```python
from build123d import *

# Parameters (mm, degrees)
SKETCH1_W           = 533.4
SKETCH1_H           = 508
SKETCH1_R           = 12.7
BOSS_EXTRUDE1_DEPTH = 152.4
BOSS_EXTRUDE2_DEPTH = 660.4
SKETCH4_OUTSIDE_W   = 729.384
SKETCH4_OUTSIDE_H   = 1034.184
CUT_EXTRUDE1_DEPTH  = 660.4
BOSS_EXTRUDE3_DEPTH = 50.8
SKETCH7_OUTSIDE_W   = 754.784
SKETCH7_OUTSIDE_H   = 1147.193
CUT_EXTRUDE2_DEPTH  = 254
CUT_EXTRUDE3_DEPTH  = 508


with BuildPart() as part:
    # Sketch1 → Boss-Extrude1 (new body)
    with BuildSketch(Plane(origin=(0, 0, 0), x_dir=(1, 0, 0), z_dir=(0, 1, 0))):
        Rectangle(SKETCH1_W, SKETCH1_H)
        with Locations(Location((-95.25, -130.175, 0), (0, 0, 90))):
            Circle(SKETCH1_R, mode=Mode.SUBTRACT)
        with Locations(Location((-95.25, 0, 0), (0, 0, 90))):
            Circle(SKETCH1_R, mode=Mode.SUBTRACT)
        with Locations(Location((-95.25, 130.175, 0), (0, 0, 90))):
            Circle(SKETCH1_R, mode=Mode.SUBTRACT)
        with Locations(Location((95.25, -130.175, 0), (0, 0, 90))):
            Circle(SKETCH1_R, mode=Mode.SUBTRACT)
        with Locations(Location((95.25, 0, 0), (0, 0, 90))):
            Circle(SKETCH1_R, mode=Mode.SUBTRACT)
        with Locations(Location((95.25, 130.175, 0), (0, 0, 90))):
            Circle(SKETCH1_R, mode=Mode.SUBTRACT)
    extrude(amount=BOSS_EXTRUDE1_DEPTH)

    # Sketch3 → Boss-Extrude2 (add)
    with BuildSketch(Plane(origin=(0, 152.4, 0), x_dir=(1, 0, 0), z_dir=(0, 1, 0))):
        Polygon((-266.7, 254), (-266.7, -254), (-165.1, -254), (165.1, -254), (266.7, -254), (266.7, 254), align=None)
    extrude(amount=BOSS_EXTRUDE2_DEPTH)

    # Sketch4 outside → Cut-Extrude1 (cut)
    with BuildSketch(Plane(origin=(266.7, 0, 0), x_dir=(0, 0, -1), z_dir=(1, 0, 0))):
        with Locations((0, 406.4)):
            Rectangle(SKETCH4_OUTSIDE_W, SKETCH4_OUTSIDE_H)
        with BuildLine():
            Line((254, 669.23901778), (254, 812.8))
            Line((254, 812.8), (228.6, 812.8))
            Line((228.6, 812.8), (31.606344145, 168.462784922))
            Line((31.606344145, 168.462784922), (-254, 168.462784922))
            ThreePointArc((-254, 168.462784922), (-243.936587472, 127.409322416), (-202.883124967, 117.345909888))
            Line((-202.883124967, 117.345909888), (-165.988990497, 0))
            Line((-165.988990497, 0), (165.353024922, 0))
            Line((165.353024922, 0), (228.6, 108.732858548))
            Line((228.6, 108.732858548), (254, 669.23901778))
        make_face(mode=Mode.SUBTRACT)
    extrude(amount=-CUT_EXTRUDE1_DEPTH, mode=Mode.SUBTRACT)

    # Sketch6 → Boss-Extrude3 (add)
    with BuildSketch(Plane.ZY.offset(266.7)):
        with BuildLine():
            Line((254, 168.462784922), (-31.606344145, 168.462784922))
            Line((-31.606344145, 168.462784922), (-93.174683572, 369.843749152))
            ThreePointArc((-93.174683572, 369.843749152), (37.15276036, 257.574854495), (204.490495991, 217.72978475))
            ThreePointArc((204.490495991, 217.72978475), (239.484222443, 203.385658011), (254, 168.462784922))
        make_face()
    boss_extrude3 = extrude(amount=-BOSS_EXTRUDE3_DEPTH)

    # Mirror1: Boss-Extrude3 across plane
    add(boss_extrude3.mirror(Plane.ZY))

    # Sketch7 outside → Cut-Extrude2 (cut)
    with BuildSketch(Plane(origin=(0, 5.563381647, 18.197001427), x_dir=(1, 0, 0), z_dir=(0, 0.29237170472274066, 0.9563047559630343))):
        with Locations((0, 388.6425)):
            Rectangle(SKETCH7_OUTSIDE_W, SKETCH7_OUTSIDE_H)
        with BuildLine():
            Line((-266.7, 380.92497735), (-209.55, 609.52497735))
            ThreePointArc((-209.55, 609.52497735), (-188.66895271, 653.395441882), (-152.4, 685.72497735))
            ThreePointArc((-152.4, 685.72497735), (-95.710918301, 736.501940936), (-63.5, 805.454161765))
            ThreePointArc((-63.5, 805.454161765), (-45.688148209, 833.291148022), (-14.465061194, 844.120677346))
            Line((-14.465061194, 844.120677346), (14.465061194, 844.120677346))
            ThreePointArc((14.465061194, 844.120677346), (45.688148209, 833.291148022), (63.5, 805.454161765))
            ThreePointArc((63.5, 805.454161765), (95.710918301, 736.501940936), (152.4, 685.72497735))
            ThreePointArc((152.4, 685.72497735), (188.66895271, 653.395441882), (209.55, 609.52497735))
            Line((209.55, 609.52497735), (266.7, 380.92497735))
            Line((266.7, 380.92497735), (266.7, -48.530484117))
            Line((266.7, -48.530484117), (-266.7, -48.530484117))
            Line((-266.7, -48.530484117), (-266.7, 380.92497735))
        make_face(mode=Mode.SUBTRACT)
    extrude(amount=-CUT_EXTRUDE2_DEPTH, mode=Mode.SUBTRACT)

    # Sketch10 → Cut-Extrude3 (cut)
    with BuildSketch(Plane.XY.offset(254)):
        with BuildLine():
            Line((-266.7, 168.462784922), (-387.417771375, 168.462784922))
            Line((-387.417771375, 168.462784922), (-387.417771375, 0))
            Line((-387.417771375, 0), (-155.638931275, 0))
            ThreePointArc((-155.638931275, 0), (-169.876966254, 49.659931769), (-208.265044728, 84.231392461))
            ThreePointArc((-208.265044728, 84.231392461), (-248.469302502, 118.725084742), (-266.7, 168.462784922))
        make_face()
        with BuildLine():
            Line((387.417771375, 0), (155.638931275, 0))
            ThreePointArc((155.638931275, 0), (169.876966254, 49.659931769), (208.265044728, 84.231392461))
            ThreePointArc((208.265044728, 84.231392461), (248.469302502, 118.725084742), (266.7, 168.462784922))
            Line((266.7, 168.462784922), (387.417771375, 168.462784922))
            Line((387.417771375, 168.462784922), (387.417771375, 0))
        make_face()
    extrude(amount=-CUT_EXTRUDE3_DEPTH, mode=Mode.SUBTRACT)


solid = part.part
```
Design review of the part built by this model. Coordinates are the model's own, in mm. A direction names the side the tool comes from. Give positions to 0.01 mm unless a question says otherwise; leave off trailing zeros. Order: outer loops, then holes, each group sorted by start corner. A loop starts at its lowest first (then second) coordinate and runs counter-clockwise, first axis right, second up. Notation, with made-up numbers: (10, 24.25) -> (24, 24.25) arc R21 cw to (24, 58.25) -> close; hole circle Ø8 at (-3, -1). An arc over 180 degrees is marked (long way). Write each question's results on one line, items separated by ' | '. Start each with the question number.
Q1. Add section C-C on z = 0. Give the boundary of the cut face in (x, y).
Q2. Wall thickness on L1, parallel to X at y = 48, z = 0; L2, parallel to Z at x = 95.25, y = 60.5 (3 decimals); L3, parallel to Z at x = -95.25, y = 50.5 (3 decimals): over which ranges is each line inside the solid? List them lowest first. Write a range as from..to.
Q3. Add section A-A on y = 49. Give the boundary of the cut face in (x, z) (3 decimals).
Q4. Add section D-D on y = 308. Give the boundary of the cut face in (x, z), and give its area (3 significant figures).
Q5. Mouldability with a two-part tool opening along Z and no side actions: class faces 1 (the flat face through (215.9, 225, 56)), 2 (the flat face through (-95, 152.4, -130)), 3 (the flat face through (-0.203, 808.972, -241.122)) as +Z half, -Z half, draft (parallel to the pull), parting line (faces both ways), or undercut.
Q6. Machinability: for faces 4 (the flat face through (95, 152.4, -130)), 5 (the cylindrical face through (-248.04, 118.11, 14.74)), which of the approach directions +Z, -Z, +X, -X, +Y, -Y give a long, thin tool a straight path to every point of the face, cutting with its end or side? Answer none if there is none.
Q7. Add section B-B on x = -95.25. Give the boundary of the cut face in (y, z) (3 decimals).
Q8. For pin 1 (6 mm diameter, centred on x = 177.5, y = 561, fed in from -Z); pin 2 (15 mm diameter, centred on x = -95.25, z = 130.175, fed in from -Y); pin 3 (15 mm diameter, centred on x = 95.25, z = 130.175, fed in from +Y), all flat-tipped, find the tip position at first contact; note any pin that passes through.
Found:
1) outline: (-266.7, 168.46) arc R104.93 ccw to (-208.27, 84.23) arc R93.72 cw to (-155.64, 0) -> (-107.95, 0) -> (-107.95, 152.4) -> (-82.55, 152.4) -> (-82.55, 0) -> (82.55, 0) -> (82.55, 152.4) -> (107.95, 152.4) -> (107.95, 0) -> (155.64, 0) arc R93.72 cw to (208.27, 84.23) arc R104.93 ccw to (266.7, 168.46) -> (266.7, 279.43) -> (215.9, 279.43) -> (215.9, 168.46) -> (-215.9, 168.46) -> (-215.9, 279.43) -> (-266.7, 279.43) -> close
2) L1: x = -168.86..-107.95, -82.55..82.55, 107.95..168.86 | L2: z = -200.544..-142.875, -117.475..-12.7, 12.7..117.475, 142.875..185.01 | L3: z = -194.728..-142.875, -117.475..-12.7, 12.7..117.475, 142.875..181.866
3) outline: (-169.468, -193.855) -> (169.468, -193.855) -> (169.468, 181.395) -> (-169.468, 181.395) -> close; hole circle Ø25.4 at (-95.25, -130.175); hole circle Ø25.4 at (-95.25, 0); hole circle Ø25.4 at (-95.25, 130.175); hole circle Ø25.4 at (95.25, -130.175); hole circle Ø25.4 at (95.25, 0); hole circle Ø25.4 at (95.25, 130.175)
4) outline: (-266.7, -237.63) -> (266.7, -237.63) -> (266.7, -37.16) -> (215.9, -37.16) -> (215.9, -74.27) -> (-215.9, -74.27) -> (-215.9, -37.16) -> (-266.7, -37.16) -> close | area: 90,900 mm2
5) face 1: draft | face 2: undercut | face 3: -Z half
6) face 4: -Y | face 5: +Z, -Z, -X, -Y
7) outline: (0, -165.353) -> (108.733, -228.6) -> (669.239, -254) -> (693.15, -254) -> (710.48, -197.318) -> (168.463, -31.606) -> (168.463, 254) -> (144.009, 254) arc R40.767 ccw to (117.346, 202.883) -> (0, 165.989) -> (0, 142.875) -> (152.4, 142.875) -> (152.4, 117.475) -> (0, 117.475) -> (0, 12.7) -> (152.4, 12.7) -> (152.4, -12.7) -> (0, -12.7) -> (0, -117.475) -> (152.4, -117.475) -> (152.4, -142.875) -> (0, -142.875) -> close
8) pin 1: stops at z = -249.23 | pin 2: stops at y = 152.4 | pin 3: stops at y = 168.46
